Autodesk Inventor part; units mm, degrees
ref_plane "YZ Plane" through (0, 0, 0) normal (1, 0, 0) x (0, 1, 0)
ref_plane "XZ Plane" through (0, 0, 0) normal (0, 1, 0) x (-1, 0, 0)
ref_plane "XY Plane" through (0, 0, 0) normal (0, 0, 1) x (1, 0, 0)
sketch "Sketch1" plane through (0, 0, 0) normal (1, 0, 0) x (0, 1, 0)
  line L0 (150, -75) -> (0, 0)
  line L1 (150, -75) -> (0, -150)
  line L2 (0, -150) -> (0, 0)
  dimension "d0" = 150
  dimension "d1" = 75
extrude "Extrusion1" add sketch "Sketch1" along normal blind 10.16
sketch "Sketch2" plane through (10.16, 0, 0) normal (1, 0, 0) x (0, 0, -1)
  point P0 (0, 0)
fillet "Fillet1" radius 19.05 1 edges at (5.08, 150, -75)
sketch "Sketch3" plane through (10.16, 0, 0) normal (1, 0, 0) x (0, 0, -1)
  arc A0 (92.0388, 115.9223) -> (57.9612, 115.9223) centre (75, 107.4029) ccw
  circle A1 centre (75, 107.4029) radius 15
  circle A2 centre (75, 107.4029) radius 10
  line L0 (75, 122.4029) -> (75, 117.4029)
  line L1 (75, 97.4029) -> (75, 92.4029)
  line L2 (85.6066, 118.0095) -> (82.0711, 114.474)
  line L3 (67.9289, 100.3318) -> (64.3934, 96.7963)
  point P0 (0, 0)
  dimension "d5" = 30
  dimension "d34" = 20
  dimension "d35" = 45
  dimension "d36" = 45
sketch "Sketch4" plane through (10.16, 0, 0) normal (1, 0, 0) x (0, 0, -1)
  line L0 (22.8055, 14.0945) -> (60.9055, 90.2945)
  line L1 (57.9612, 115.9223) -> (0, 0)
  line L2 (22.8055, 14.0945) -> (60.9055, 14.0945)
  line L3 (60.9055, 14.0945) -> (60.9055, 90.2945)
  line L4 (0, 0) -> (150, 0) construction
  line L5 (0, 0) -> (150, 0) construction
  arc A0 (92.0388, 115.9223) -> (57.9612, 115.9223) centre (75, 107.4029) ccw construction
  line L6 (75, 126.4529) -> (75, 0) construction
  line L7 (127.1945, 14.0945) -> (89.0945, 90.2945)
  line L8 (127.1945, 14.0945) -> (89.0945, 14.0945)
  line L9 (89.0945, 14.0945) -> (89.0945, 90.2945)
  dimension "d8" = 76.2
  dimension "d11" = 14.0945
  dimension "d12" = 14.0945
  dimension "d13" = 14.0945
extrude "Extrusion3" cut sketch "Sketch4" against normal through all
fillet "Fillet2" radius 5 1 edges at (5.08, 14.0945, -127.1945)
fillet "Fillet3" radius 5 2 edges at (5.08, 14.0945, -89.0945) (5.08, 90.2945, -89.0945)
fillet "Fillet4" radius 5 3 edges at (5.08, 14.0945, -60.9055) (5.08, 90.2945, -60.9055) (5.08, 14.0945, -22.8055)
sketch "Sketch6" plane through (0, 0, -150) normal (0, -1, 0) x (1, 0, 0)
  line L0 (10.16, 150) -> (10.16, 0) construction
  line L1 (10.16, 75) -> (0, 75) construction
  line L2 (0, 65) -> (0, 85) construction
  line L3 (7.493, 126.597) -> (2.667, 126.597)
  line L4 (2.667, 126.597) -> (2.667, 107.801)
  line L5 (2.667, 107.801) -> (7.493, 107.801)
  line L6 (7.493, 107.801) -> (7.493, 126.597)
  line L7 (0, 150) -> (0, 0)
  line L8 (0, 150) -> (10.16, 150)
  line L9 (7.493, 84.398) -> (2.667, 84.398)
  line L10 (2.667, 84.398) -> (2.667, 65.602)
  line L11 (2.667, 65.602) -> (7.493, 65.602)
  line L12 (7.493, 65.602) -> (7.493, 84.398)
  line L13 (7.493, 23.403) -> (2.667, 23.403)
  line L14 (2.667, 23.403) -> (2.667, 42.199)
  line L15 (2.667, 42.199) -> (7.493, 42.199)
  line L16 (7.493, 42.199) -> (7.493, 23.403)
  dimension "d22" = 4.826
  dimension "d23" = 2.667
  dimension "d24" = 2.667
  dimension "d25" = 18.796
  dimension "d26" = 23.403
  dimension "d27" = 18.796
  dimension "d29" = 4.826
  dimension "d30" = 2.667
  dimension "d31" = 2.667
  dimension "d41" = 23.403
extrude "Extrusion5" add sketch "Sketch6" along normal blind 10.16
extrude "Extrusion7" cut sketch "Sketch3" against normal through all
sketch "Sketch7" plane through (10.16, 0, 0) normal (1, 0, 0) x (0, 0, -1)
  circle A0 centre (75, 107.4029) radius 15
  line L0 (60, 107.4029) -> (60, 119.1461)
  arc A1 (92.0388, 115.9223) -> (57.9612, 115.9223) centre (75, 107.4029) ccw
  line L1 (90, 107.4029) -> (90, 119.1461)
  arc A2 (90, 107.4029) -> (60, 107.4029) centre (75, 107.4029) ccw
  arc A3 (90, 119.1461) -> (60, 119.1461) centre (75, 107.4029) ccw
  point P0 (0, 0)
extrude "Extrusion8" cut sketch "Sketch7" against normal through all contours A0 L0 A1 L1
equation "\"d11\" = d13"
equation "\"d12\" = d11"
equation "\"d23\" = d24"
equation "\"d26\" = d41"
equation "\"d27\" = d25"
equation "\"d29\" = d22"
equation "\"d30\" = d23"
properties part number "spool holder arm side1" material "PLA"
Verification items for the finished model (mm, model axes). A direction names the side the tool comes from. Give positions to 0.01 mm unless a question says otherwise; leave off trailing zeros. Loops run counter-clockwise (first coordinate to the right, second up) from the corner with the lowest first, then second, coordinate; pieces in that order, holes last.
1. Tool access check on faces 1 (the flat face through (7.493, -5, -117)), 2 (the flat face through (5, -5, -107.801)), 3 (the flat face through (2.667, -5, -117)), 4 (the cylindrical face through (5.009, 16.406, -26.68)). Record the directions out of +Z, -Z, +X, -X, +Y, -Y that give a thin tool (end or side, any length) a straight path to the whole face; none if there is none.
Derived:
face 1: +Z, -Z, +X, -Y
face 2: +X, -X, -Y
face 3: +Z, -Z, -X, -Y
face 4: +X, -X
2. Release check for a two-part mould opening along Z. For faces 5 (the cylindrical face through (5.151, 117.608, -58.914)), 6 (the flat face through (5, -10.16, -117)), 7 (the flat face through (5, 58.8, -120.6)), 8 (the flat face through (5, 44, -89.094)) record: +Z half, -Z half, draft (parallel to the pull), parting line (faces both ways), or undercut.
Derived:
face 5: +Z half
face 6: draft
face 7: -Z half
face 8: undercut
3. Cross-section at A-A on x = 5. Count the separate pieces of the cut face and the enclosed holes in it, and give its area (3 significant figures).
Derived:
separate pieces: 1
enclosed holes: 2
area: 7,920 mm2
4. Material ranges on probe 1 along Z at (x, y) = (0.5, 64); probe 2 along Z at (x, y) = (3.75, 40.5); probe 3 along Y at (x, z) = (5.5, -116.5), recorded low to high.
Derived:
probe 1: z = -118 to -102.24, -89.09 to -60.91, -47.76 to -32
probe 2: z = -129.75 to -113.99, -89.09 to -60.91, -36.01 to -20.25
probe 3: y = -10.16 to 14.09, 35.48 to 67
5. Go/stop test with flat-tipped pins: P1, Ø5, axis at x = 3, y = 66.5, coming from the -Z side; P2, Ø6, axis at x = 8, y = 76, coming from the -Z side; P3, Ø3, axis at y = -3, z = -76, coming from the +X side. Record where each tip stops, or that it passes through.
Derived:
P1: stops at z = -118
P2: stops at z = -113.5
P3: stops at x = 7.49
6. Cross-section at B-B on y = 104. Record the cut outline in (x, z).
Derived:
outline: (0, -98) - (10.16, -98) - (10.16, -89.61) - (0, -89.61) - close; (0, -60.39) - (10.16, -60.39) - (10.16, -52) - (0, -52) - close
7. Cross-section at D-D on z = -75. Record the cut outline in (x, y).
Derived:
outline: (0, 0) - (2.67, 0) - (2.67, -10.16) - (7.49, -10.16) - (7.49, 0) - (10.16, 0) - (10.16, 92.4) - (0, 92.4) - close
8. Cross-section at C-C on z = -101. Record the cut outline in (x, y).
Derived:
outline: (0, 0) - (10.16, 0) - (10.16, 14.09) - (0, 14.09) - close; (0, 66.48) - (10.16, 66.48) - (10.16, 98) - (0, 98) - close
